Autodesk Inventor part; units mm, degrees
ref_plane "YZ Plane" through (0, 0, 0) normal (1, 0, 0) x (0, 1, 0)
ref_plane "XZ Plane" through (0, 0, 0) normal (0, 1, 0) x (-1, 0, 0)
ref_plane "XY Plane" through (0, 0, 0) normal (0, 0, 1) x (1, 0, 0)
sketch "Szkic1" plane through (0, 0, 0) normal (0, 0, 1) x (1, 0, 0)
  line L0 (0, 0) -> (10, 0)
  line L1 (10, 0) -> (-10, 0)
  line L2 (-10, 0) -> (-10, 65)
  line L3 (10, 0) -> (10, 65)
  line L4 (-10, 65) -> (-10, 53)
  line L5 (10, 65) -> (7, 65)
  line L6 (-10, 65) -> (-7, 65)
  line L7 (4, 53) -> (-4, 53)
  line L8 (-7, 65) -> (-4, 53)
  line L9 (4, 53) -> (7, 65)
  point P0 (2, 53)
  dimension "d2" = 65
  dimension "d4" = 12
  dimension "d5" = 6
  dimension "d17" = 3
  dimension "d18" = 3
revolve "Obrót1" add sketch "Szkic1" angle 360 about axis through (10, 0, 0) along (-1, 0, 0)
sketch "Szkic2" plane through (10, 0, 0) normal (1, 0, 0) x (0, 0, -1)
  circle A0 centre (0, 0) radius 10
  dimension "d8" = 20
extrude "Wyciągnięcie proste1" cut sketch "Szkic2" against normal blind 100
properties part number "kolo"
Geometry check sheet. Reference: the model listing, model coordinates, mm. A direction names the side the tool comes from. Round coordinates to 2 decimals unless told otherwise and drop trailing zeros. Order: outer loops, then holes, each group sorted by start corner. A loop starts at its lowest first (then second) coordinate and runs counter-clockwise, first axis right, second up. Notation, with made-up numbers: M 7.25,-1 L 33.25,-1 A20 cw 33.25,27 Z; hole C 55,-5.75 d6. An arc over 180 degrees is marked long. Write item = value, one per line.
Q1. Depth check by flat-ended pin: pin 1 Ø5 at (x, z) = (6, -29.5) entering from -Y; pin 2 Ø2 at (x, z) = (6.5, -10.5) entering from +Y; pin 3 Ø1.5 at (x, y) = (-1.5, -2.5) entering from -Z. Enter the tip coordinate at first touch or a pass-through.
Answer block:
pin_1 = -59.03
pin_2 = 64.28
pin_3 = -52.97
Q2. Scan lines: line 1 (Y direction, x = -0.5, z = 0); line 2 (X direction, y = 58.5, z = 2); line 3 (X direction, y = -33.5, z = 45). Record each from-to range of solid material in increasing order.
Answer block:
line_1 = -53 to -10, 10 to 53
line_2 = -10 to -5.38, 5.38 to 10
line_3 = -10 to -4.78, 4.78 to 10
Q3. Section check D-D (x = -1.75). Enter the section's corners in (y, z).
Answer block:
outline = C 0,0 d106; hole C 0,0 d20
Q4. Section check A-A (y = 0). Enter the section's corners in (x, z).
Answer block:
outline = M -10,-65 L -7,-65 L -4,-53 L 4,-53 L 7,-65 L 10,-65 L 10,-10 L -10,-10 Z; M -10,10 L 10,10 L 10,65 L 7,65 L 4,53 L -4,53 L -7,65 L -10,65 Z
Q5. Section check C-C (x = -8.5). Enter the section's corners in (y, z).
Answer block:
outline = C 0,0 d130; hole C 0,0 d20
Q6. Release check for a two-part mould opening along Y. For faces 1 (the flat face through (10, 14, -1)), 2 (the cylindrical face through (-8.48, 62, 19.52)), 3 (the cylindrical face through (0.14, -9.76, 2.17)) record: released by +Y, released by -Y, zero draft, split by the parting line, or undercut.
Answer block:
face_1 = zero draft
face_2 = split by the parting line
face_3 = undercut
Q7. Set-up check for faces 4 (the cylindrical face through (8.48, 62, -19.52)), 5 (the conical face through (-4.188, -11.652, 52.472)): record each of +Z, -Z, +X, -X, +Y, -Y from which the full face is reachable in a straight line by a thin tool's end or side.
Answer block:
face_4 = +X, -X
face_5 = none
